```python
from build123d import *

# Parameters (mm, degrees)
F0_W        = 88.9
F0_H        = 152.4
F1_DEPTH    = 6.35
F2_DEPTH    = 25.4
F3_DEPTH    = 50.8
F4_C1_SIZE2 = 12.7
F4_C1_SIZE  = 7.3323484187
F4_C2_SIZE2 = 12.7
F4_C2_SIZE  = 7.3323484187
F4_C3_SIZE2 = 7.3323484187
F4_C3_SIZE  = 12.7
F4_C4_SIZE2 = 12.7
F4_C4_SIZE  = 7.3323484187


with BuildPart() as f1:
    # F0 (on Top) → F1 (new body)
    with BuildSketch(Plane.XY):
        with Locations((-31.1787627001, 11.3253805135)):
            Rectangle(F0_W, F0_H)
        Polygon((-69.2787627001, 43.0753805135), (-69.2787627001, 81.1753805135), (-31.1787627001, 81.1753805135), (6.9212372999, 81.1753805135), (6.9212372999, -20.4246194865), (6.9212372999, -58.5246194865), (-31.1787627001, -58.5246194865), (-69.2787627001, -58.5246194865), align=None, mode=Mode.SUBTRACT)
    extrude(amount=F1_DEPTH)

    # F0 (on Top) → F2 (join)
    with BuildSketch(Plane.XY):
        with BuildLine():
            Line((6.9212372999, 81.1753805135), (-31.1787627001, 81.1753805135))
            Line((-31.1787627001, 81.1753805135), (-31.1787627001, 55.7753805135))
            ThreePointArc((-31.1787627001, 55.7753805135), (-34.898506579, 46.7951243925), (-43.8787627001, 43.0753805135))
            Line((-43.8787627001, 43.0753805135), (-69.2787627001, 43.0753805135))
            Line((-69.2787627001, 43.0753805135), (-69.2787627001, -58.5246194865))
            Line((-69.2787627001, -58.5246194865), (-31.1787627001, -58.5246194865))
            Line((-31.1787627001, -58.5246194865), (-31.1787627001, -33.0056861837))
            ThreePointArc((-31.1787627001, -33.0056861837), (-26.8234670857, -23.4319769383), (-16.7447613275, -20.4246194865))
            Line((-16.7447613275, -20.4246194865), (6.9212372999, -20.4246194865))
            Line((6.9212372999, -20.4246194865), (6.9212372999, 81.1753805135))
        make_face()
    extrude(amount=F2_DEPTH)

    # F0 (on Top) → F3 (join)
    with BuildSketch(Plane.XY):
        with BuildLine():
            Line((-31.1787627001, 81.1753805135), (-69.2787627001, 81.1753805135))
            Line((-69.2787627001, 81.1753805135), (-69.2787627001, 43.0753805135))
            Line((-69.2787627001, 43.0753805135), (-43.8787627001, 43.0753805135))
            ThreePointArc((-43.8787627001, 43.0753805135), (-34.898506579, 46.7951243925), (-31.1787627001, 55.7753805135))
            Line((-31.1787627001, 55.7753805135), (-31.1787627001, 81.1753805135))
        make_face()
        with BuildLine():
            Line((6.9212372999, -58.5246194865), (6.9212372999, -20.4246194865))
            Line((6.9212372999, -20.4246194865), (-16.7447613275, -20.4246194865))
            ThreePointArc((-16.7447613275, -20.4246194865), (-26.8234670857, -23.4319769383), (-31.1787627001, -33.0056861837))
            Line((-31.1787627001, -33.0056861837), (-31.1787627001, -58.5246194865))
            Line((-31.1787627001, -58.5246194865), (6.9212372999, -58.5246194865))
        make_face()
    extrude(amount=F3_DEPTH)

    # F4: chamfer of 12.7 x 7.3323484187 on 4 edges, made by hand

    # F4_c1
    f4_c1_edges = [f1.edges().sort_by_distance(p)[0] for p in [
        (-12.1287627001, -58.5246194865, 50.8),
    ]]
    f4_c1_side = f1.faces().sort_by_distance((-12.1287627001, -58.5246194865, 50.6533530316))[0]
    chamfer(f4_c1_edges, length=F4_C1_SIZE, length2=F4_C1_SIZE2, reference=f4_c1_side)

    # F4_c2
    f4_c2_edges = [f1.edges().sort_by_distance(p)[0] for p in [
        (6.9212372999, -33.1246194865, 50.8),
    ]]
    f4_c2_side = f1.faces().sort_by_distance((6.9212372999, -33.1246194865, 50.6533530316))[0]
    chamfer(f4_c2_edges, length=F4_C2_SIZE, length2=F4_C2_SIZE2, reference=f4_c2_side)

    # F4_c3
    f4_c3_edges = [f1.edges().sort_by_distance(p)[0] for p in [
        (-50.2287627001, 81.1753805135, 50.8),
    ]]
    f4_c3_side = f1.faces().sort_by_distance((-50.2287627001, 81.1753805135, 50.6533530316))[0]
    chamfer(f4_c3_edges, length=F4_C3_SIZE, length2=F4_C3_SIZE2, reference=f4_c3_side)

    # F4_c4
    f4_c4_edges = [f1.edges().sort_by_distance(p)[0] for p in [
        (-69.2787627001, 58.4592063042, 50.8),
    ]]
    f4_c4_side = f1.faces().sort_by_distance((-69.2787627001, 58.4592063042, 50.6533530316))[0]
    chamfer(f4_c4_edges, length=F4_C4_SIZE, length2=F4_C4_SIZE2, reference=f4_c4_side)


solid = f1.part
```
Source: CAD feature listing. Evaluate the final solid. Frame: model axes, mm. A direction names the side the tool comes from. Round coordinates to 2 decimals unless told otherwise and drop trailing zeros. Loops run counter-clockwise (first coordinate to the right, second up) from the corner with the lowest first, then second, coordinate; pieces in that order, holes last.
(1) Section query C-C (z = 20.5). Output: boundary loops of the cut face in (x, y), and give its area (3 significant figures).
From the geometry:
outline: (-69.28, -58.52) - (6.92, -58.52) - (6.92, 81.18) - (-69.28, 81.18) - close
area: 10,600 mm2
(2) Section query D-D (x = -67). Output: boundary loops of the cut face in (y, z).
From the geometry:
outline: (-64.87, 0) - (87.53, 0) - (87.53, 6.35) - (81.18, 6.35) - (81.18, 38.1) - (77.32, 44.78) - (43.08, 44.78) - (43.08, 25.4) - (-58.52, 25.4) - (-58.52, 6.35) - (-64.87, 6.35) - close
(3) Section query B-B (x = -54). Output: boundary loops of the cut face in (y, z).
From the geometry:
outline: (-64.87, 0) - (87.53, 0) - (87.53, 6.35) - (81.18, 6.35) - (81.18, 38.1) - (73.84, 50.8) - (43.08, 50.8) - (43.08, 25.4) - (-58.52, 25.4) - (-58.52, 6.35) - (-64.87, 6.35) - close
(4) Material intervals for probe 1 along Z at (x, y) = (-49, -50); probe 2 along Y at (x, z) = (-1, 40); probe 3 along Y at (x, z) = (-34, 9), sorted ascending.
From the geometry:
probe 1: z = 0 to 25.4
probe 2: y = -58.52 to -20.42
probe 3: y = -58.52 to 81.18
(5) Access query for faces 1 (the flat face through (-32, 12, 25.4)), 2 (the flat face through (-39, 81.175, 18)), 3 (the flat face through (6.921, -5, 21)). Directions: +Z, -Z, +X, -X, +Y, -Y. A direction counts if a zero-diameter tool reaches every point of the face in a straight line with its end or side. Return the directions, or none.
From the geometry:
face 1: +Z
face 2: +Z, +X, -X, +Y
face 3: +Z, +X, +Y, -Y
(6) Contact query for flat-ended pins moving along their axis: pin 1 Ø4 at (y, z) = (5, 23.5) entering from +X; pin 2 Ø20.5 at (y, z) = (-46.5, 42) entering from -X; pin 3 Ø16 at (x, z) = (-43.5, 26.5) entering from +Y. Output: stop coordinate, or through.
From the geometry:
pin 1: stops at x = 6.92
pin 2: stops at x = -31.18
pin 3: stops at y = 81.18
(7) Section query A-A (y = -6). Output: boundary loops of the cut face in (x, z), and give its area (3 significant figures).
From the geometry:
outline: (-75.63, 0) - (13.27, 0) - (13.27, 6.35) - (6.92, 6.35) - (6.92, 25.4) - (-69.28, 25.4) - (-69.28, 6.35) - (-75.63, 6.35) - close
area: 2,020 mm2
